```python
from build123d import *

# Parameters (mm, degrees)
F0_W     = 87.854118
F0_H     = 61.326738
F1_DEPTH = 25.4
F2_R     = 20.514038
F3_DEPTH = 25.4
F4_R     = 15.848833
F5_DEPTH = 50.8
F6_R     = 16.894941
F7_DEPTH = 76.2


with BuildPart() as f1:
    # F0 (on Front) → F1 (new body)
    with BuildSketch(Plane.XZ):
        Rectangle(F0_W, F0_H)
    extrude(amount=F1_DEPTH)

    # F2 (on face) → F3 (join)
    with BuildSketch(Plane.XZ.offset(25.4)):
        Circle(F2_R)
    extrude(amount=F3_DEPTH)

    # F4 (on Front) → F5 (cut)
    with BuildSketch(Plane.XZ):
        Circle(F4_R)
    extrude(amount=-F5_DEPTH, mode=Mode.SUBTRACT)

    # F6 (on face) → F7 (cut)
    with BuildSketch(Plane.XZ.offset(50.8)):
        Circle(F6_R)
    extrude(amount=-F7_DEPTH, mode=Mode.SUBTRACT)


solid = f1.part
```
Geometry: final body of the model. Coordinates: model frame, mm. A direction names the side the tool comes from. Give positions to 0.01 mm unless a question says otherwise; leave off trailing zeros. Loops run counter-clockwise (first coordinate to the right, second up) from the corner with the lowest first, then second, coordinate; pieces in that order, holes last. Notation, with made-up numbers: (80.25, 50.5) -> (94.25, 50.5) arc R22 ccw to (94.25, 58.5) -> close; hole circle Ø1 at (51, 21.25). An arc over 180 degrees is marked (long way). Use one line per item in the form item = value.
Item 1: Line query: probe 1 along Z at (x, y) = (0, -20); probe 2 along Z at (x, y) = (0, -40); probe 3 along Y at (x, z) = (-22, 10). Output: solid intervals per line, ascending.
A:
probe_1 = -30.66 to -16.89, 16.89 to 30.66
probe_2 = -20.51 to -16.89, 16.89 to 20.51
probe_3 = -25.4 to 0
Item 2: Draft query along Z for faces 1 (the face through (15.607, -25.756, -6.471)), 2 (the face through (-1, -13, -30.663)), 3 (the face through (-1, -13, 30.663)), 4 (the face through (-10, 0, 14)). Return one class per face: pulls with the +Z half, pulls with the -Z half, needs draft (parallel to the pull), parting line crosses it, or undercut.
A:
face_1 = undercut
face_2 = pulls with the -Z half
face_3 = pulls with the +Z half
face_4 = needs draft
Item 3: Section query D-D on x = 32.5. Output: boundary loops of the cut face in (y, z), and give its area (3 significant figures).
A:
outline = (-25.4, -30.66) -> (0, -30.66) -> (0, 30.66) -> (-25.4, 30.66) -> close
area = 1,560 mm^2
Item 4: Section query C-C on y = -4. Output: boundary loops of the cut face in (x, z).
A:
outline = (-43.93, -30.66) -> (43.93, -30.66) -> (43.93, 30.66) -> (-43.93, 30.66) -> close; hole circle Ø33.79 at (0, 0)
Item 5: Pin query (flat end, axial travel): P1, Ø6, axis at x = 12, y = -34.5, coming from the -Z side; P2, Ø6, axis at y = -27.5, z = -18, coming from the -X side; P3, Ø10, axis at x = -33, z = -16.5, coming from the -Y side; P4, Ø1.5, axis at y = -35, z = 17, coming from the -X side. Return the tip coordinate at first contact, or that it passes through.
A:
P1 = -18.43
P2 = -43.93
P3 = -25.4
P4 = -12.52
Item 6: Section query B-B on z = 0. Output: boundary loops of the cut face in (x, y), and give its area (3 significant figures).
A:
outline = (-43.93, -25.4) -> (-20.51, -25.4) -> (-20.51, -50.8) -> (-16.89, -50.8) -> (-16.89, 0) -> (-43.93, 0) -> close; (16.89, -50.8) -> (20.51, -50.8) -> (20.51, -25.4) -> (43.93, -25.4) -> (43.93, 0) -> (16.89, 0) -> close
area = 1,560 mm^2
Item 7: Section query A-A on x = 0. Output: boundary loops of the cut face in (y, z).
A:
outline = (-50.8, -20.51) -> (-25.4, -20.51) -> (-25.4, -30.66) -> (0, -30.66) -> (0, -16.89) -> (-50.8, -16.89) -> close; (-50.8, 16.89) -> (0, 16.89) -> (0, 30.66) -> (-25.4, 30.66) -> (-25.4, 20.51) -> (-50.8, 20.51) -> close
Item 8: Access query for faces 5 (the face through (-43.927, -13, 0)), 6 (the face through (-20, -25.4, 7)). Directions: +Z, -Z, +X, -X, +Y, -Y. A direction counts if a zero-diameter tool reaches every point of the face in a straight line with its end or side. Return the directions, or none.
A:
face_5 = +Z, -Z, -X, +Y, -Y
face_6 = -Y
